The model under review builds one solid part; all positions refer to its coordinate system, in mm. A direction names the side the tool comes from. Round coordinates to 2 decimals unless told otherwise and drop trailing zeros. Order: outer loops, then holes, each group sorted by start corner. A loop starts at its lowest first (then second) coordinate and runs counter-clockwise, first axis right, second up. Notation, with made-up numbers: M -26.75,65 L -11.75,65 A17 ccw -11.75,72 Z; hole C 1,86 d10. An arc over 180 degrees is marked long. Answer as CSV lines item,"result". Start each with the question number.
from build123d import *

# Parameters (mm, degrees)
SKETCH1_W                       = 38.1
SKETCH1_H                       = 38.1
BOSS_EXTRUDE1_DEPTH             = 6.35
F_8_32_TAPPED_HOLE1_D           = 3.4544
F_8_32_TAPPED_HOLE1_CSINK_D     = 5.4356
F_8_32_TAPPED_HOLE1_CSINK_ANGLE = 100
SKETCH6_W                       = 6
SKETCH6_H                       = 6
CUT_EXTRUDE1_DEPTH              = 55.254423783


with BuildPart() as part:
    # Sketch1 → Boss-Extrude1 (new body)
    with BuildSketch(Plane(origin=(0, 0, 0), x_dir=(1, 0, 0), z_dir=(0, 1, 0))):
        with Locations((19.05, 19.05)):
            Rectangle(SKETCH1_W, SKETCH1_H)
    extrude(amount=BOSS_EXTRUDE1_DEPTH)

    # #8-32 Tapped Hole1 (through all)
    with Locations(Plane(origin=(0, 6.35, 0), x_dir=(1, 0, 0), z_dir=(0, 1, 0))):
        with Locations((31.75, 31.75), (6.35, 31.75), (6.35, 6.35), (31.75, 6.35)):
            CounterSinkHole(F_8_32_TAPPED_HOLE1_D / 2, F_8_32_TAPPED_HOLE1_CSINK_D / 2, counter_sink_angle=F_8_32_TAPPED_HOLE1_CSINK_ANGLE)

    # Sketch5 → M18 Clearance Hole1 (revolve, cut)
    with BuildSketch(Plane(origin=(19.05, 6.35, -19.05), x_dir=(0, 0, 1), z_dir=(1, 0, 0))):
        Polygon((0, 0), (0, 6.35), (10, 6.35), (10, 0.020977491), (10.025, 0), align=None)
    revolve(axis=Axis((19.05, 12.7, -19.05), (0, -1, 0)), mode=Mode.SUBTRACT)

    # Sketch6 → Cut-Extrude1 (cut, through all)
    with BuildSketch(Plane(origin=(0, 6.35, 0), x_dir=(1, 0, 0), z_dir=(0, 1, 0))):
        with Locations((10.55, 19.05)):
            Rectangle(SKETCH6_W, SKETCH6_H)
    extrude(amount=-CUT_EXTRUDE1_DEPTH, mode=Mode.SUBTRACT)


solid = part.part
Item 1: Consider section B-B (x = 19.05). State the section outline as (y, z) points (3 decimals).
Item 2: Consider section D-D (y = 1.5). State the section outline as (x, z) points.
Item 3: Consider section C-C (z = -6.35). State the section outline as (x, y) points, and give its area (3 significant figures).
Item 4: Consider section A-A (z = -19.05). State the section outline as (x, y) points (3 decimals), and give its area (3 significant figures).
Item 5: Tool access review of faces 5 (the flat face through (38.1, 3, -19)), 6 (the flat face through (9, 3, -22.05)): name each direction out of +Z, -Z, +X, -X, +Y, -Y from which nothing blocks a thin tool from reaching the whole face with its end or side.
Item 6: Wall thickness on probe 1 along Z at (x, y) = (6.35, 2.85); probe 2 along X at (y, z) = (1.95, -6.35); probe 3 along X at (y, z) = (2.25, -33): over which ranges is each line inside the solid? List them lowest first. Write a range as [from, to].
Item 7: For pin 1 (4 mm diameter, centred on x = 31.75, z = -31.75, fed in from +Y), flat-tipped, find the tip position at first contact; note if it passes through.
Item 8: The part is to be moulded in two halves that separate along Z. For faces 1 (the flat face through (10, 6.35, -28)), 2 (the cylindrical face through (6.724, 2.721, -30.064)), 3 (the flat face through (19, 3, -38.1)), 4 (the cylindrical face through (30.155, 2.721, -5.688)), say which applies: +Z half, -Z half, draft (parallel to the pull), parting line (faces both ways), or undercut.
Reported:
1,outline,"M 0,-38.1 L 6.35,-38.1 L 6.35,-29.075 L 6.329,-29.05 L 0,-29.05 Z; M 0,-9.05 L 6.329,-9.05 L 6.35,-9.025 L 6.35,0 L 0,0 Z"
2,outline,"M 0,-38.1 L 38.1,-38.1 L 38.1,0 L 0,0 Z; hole C 6.35,-31.75 d3.45; hole C 6.35,-6.35 d3.45; hole M 7.55,-22.05 L 9.51,-22.05 A10 ccw long 9.51,-16.05 L 7.55,-16.05 Z; hole C 31.75,-31.75 d3.45; hole C 31.75,-6.35 d3.45"
3,outline,"M 0,0 L 4.62,0 L 4.62,5.52 L 3.63,6.35 L 0,6.35 Z; M 8.08,0 L 30.02,0 L 30.02,5.52 L 29.03,6.35 L 9.07,6.35 L 8.08,5.52 Z; M 33.48,0 L 38.1,0 L 38.1,6.35 L 34.47,6.35 L 33.48,5.52 Z"
3,area,"196 mm²"
4,outline,"M 0,0 L 7.55,0 L 7.55,6.35 L 0,6.35 Z; M 29.05,0 L 38.1,0 L 38.1,6.35 L 29.075,6.35 L 29.05,6.329 Z"
4,area,"105 mm²"
5,face 5,"+Z, -Z, +X, +Y, -Y"
5,face 6,"+Y, -Y"
6,probe 1,"z = [-38.1, -33.48], [-30.02, -8.08], [-4.62, 0]"
6,probe 2,"x = [0, 4.62], [8.08, 30.02], [33.48, 38.1]"
6,probe 3,"x = [0, 5.16], [7.54, 30.56], [32.94, 38.1]"
7,pin 1,"stops at y = 5.75"
8,face 1,"draft"
8,face 2,"undercut"
8,face 3,"-Z half"
8,face 4,"undercut"
